Source: CAD feature listing. Evaluate the final solid. Frame: model axes, mm. A direction names the side the tool comes from. Coordinates: 2 decimals unless noted, no trailing zeros. Order: outer loops, then holes, each group sorted by start corner. A loop starts at its lowest first (then second) coordinate and runs counter-clockwise, first axis right, second up.
```python
from build123d import *

# Parameters (mm, degrees)
SKETCH1_R           = 2.5
BOSS_EXTRUDE1_DEPTH = 10
SKETCH2_R           = 4.8
BOSS_EXTRUDE2_DEPTH = 1.12
FILLET2_R           = 0.4


with BuildPart() as part:
    # Sketch1 → Boss-Extrude1 (new body)
    with BuildSketch(Plane(origin=(0, 0, 0), x_dir=(1, 0, 0), z_dir=(0, 1, 0))):
        with Locations(Location((0, 0, 0), (0, 0, 270))):
            Circle(SKETCH1_R)
    extrude(amount=BOSS_EXTRUDE1_DEPTH)

    # Sketch2 → Boss-Extrude2 (add)
    with BuildSketch(Plane(origin=(0, 10, 0), x_dir=(1, 0, 0), z_dir=(0, 1, 0))):
        with Locations(Location((0, 0, 0), (0, 0, 270))):
            Circle(SKETCH2_R)
    extrude(amount=BOSS_EXTRUDE2_DEPTH)

    # Fillet2
    fillet2_edges = [part.edges().sort_by_distance(p)[0] for p in [
        (0, 11.12, -4.8),
    ]]
    fillet(fillet2_edges, radius=FILLET2_R)


solid = part.part
```
1. Ray query, line 1 (X direction, y = 5.5, z = 0); line 2 (Y direction, x = 2.5, z = -1); line 3 (Z direction, x = 2.25, y = 2). Return the intervals inside material, ascending.
Findings:
line 1: x = -2.5 to 2.5
line 2: y = 10 to 11.12
line 3: z = -1.09 to 1.09
2. Section query D-D on y = 10.5. Return loops of the section in (x, z), plus the area to 3 significant figures.
Findings:
outline: circle Ø9.6 at (0, 0)
area: 72.4 mm2
3. Section query B-B on x = 0. Return loops of the section in (y, z).
Findings:
outline: (0, -2.5) - (10, -2.5) - (10, -4.8) - (10.72, -4.8) arc R0.4 ccw to (11.12, -4.4) - (11.12, 4.4) arc R0.4 ccw to (10.72, 4.8) - (10, 4.8) - (10, 2.5) - (0, 2.5) - close
4. Pin query (flat end, axial travel): P1, Ø3, axis at x = -1.5, y = 7.5, coming from the -Z side; P2, Ø4, axis at y = 3, z = 1.5, coming from the -X side; P3, Ø2, axis at x = 2.5, y = 8, coming from the +Z side. Return the tip coordinate at first contact, or that it passes through.
Findings:
P1: stops at z = -2.5
P2: stops at x = -2.5
P3: stops at z = 2
5. Section query A-A on z = 0. Return loops of the section in (x, y).
Findings:
outline: (-4.8, 10) - (-2.5, 10) - (-2.5, 0) - (2.5, 0) - (2.5, 10) - (4.8, 10) - (4.8, 10.72) arc R0.4 ccw to (4.4, 11.12) - (-4.4, 11.12) arc R0.4 ccw to (-4.8, 10.72) - close
6. Access query for faces 1 (the face through (0, 0, 0)), 2 (the face through (-2, 10, 2)). Directions: +Z, -Z, +X, -X, +Y, -Y. A direction counts if a zero-diameter tool reaches every point of the face in a straight line with its end or side. Return the directions, or none.
Findings:
face 1: +Z, -Z, +X, -X, -Y
face 2: -Y
7. Section query C-C on y = 8.5. Return loops of the section in (x, z).
Findings:
outline: circle Ø5 at (0, 0)
